Part model, mm, in its own coordinate system. Face numbers are marked on the shaded views. A direction names the side the tool comes from. Round coordinates to 2 decimals unless told otherwise and drop trailing zeros. Loops run counter-clockwise (first coordinate to the right, second up) from the corner with the lowest first, then second, coordinate; pieces in that order, holes last. Notation, with made-up numbers: M 43,29.25 L 89,29.25 A25 ccw 89,65.25 Z; hole C 46,67.5 d5. An arc over 180 degrees is marked long. Put each result on its own line as item: value. Start each with the question number.
```python
from build123d import *

# Parameters (mm, degrees)
SKETCH1_W           = 6.35
SKETCH1_H           = 19.05
SKETCH1_R           = 2.159
BOSS_EXTRUDE1_DEPTH = 19.05
SKETCH2_W           = 14.5796
SKETCH2_H           = 19.05
BOSS_EXTRUDE2_DEPTH = 19.05
SKETCH3_R           = 22.352
CUT_EXTRUDE1_DEPTH  = 2.57175
CUT_EXTRUDE2_REACH  = 34.996
SKETCH4_W           = 3.175
SKETCH4_H           = 19.05
CUT_EXTRUDE3_REACH  = 33.27
SKETCH6_W           = 6.35
SKETCH6_H           = 1.5875
FILLET2_R           = 0.254
FILLET3_START       = -15.6210001
FILLET3_DEPTH       = 5.918275981
FILLET3_START_2     = 9
FILLET3_2_DEPTH     = 8
CUT_EXTRUDE4_START  = -14.5796
CUT_EXTRUDE4_DEPTH  = 14.5796


with BuildPart() as part:
    # Sketch1 → Boss-Extrude1 (new body)
    with BuildSketch(Plane.XY):
        with Locations((3.175, 9.525)):
            Rectangle(SKETCH1_W, SKETCH1_H)
        with Locations(Location((3.175, 14.3764, 0), (0, 0, 180))):
            Circle(SKETCH1_R, mode=Mode.SUBTRACT)
        with Locations(Location((3.175, 4.6736, 0), (0, 0, 180))):
            Circle(SKETCH1_R, mode=Mode.SUBTRACT)
    extrude(amount=BOSS_EXTRUDE1_DEPTH)

    # Sketch2 → Boss-Extrude2 (add)
    with BuildSketch(Plane.ZY):
        with Locations((11.7602, 9.525)):
            Rectangle(SKETCH2_W, SKETCH2_H)
    extrude(amount=BOSS_EXTRUDE2_DEPTH)

    # Sketch3 → Cut-Extrude1 (cut, symmetric)
    with BuildSketch(Plane(origin=(0, 0, 13.31595), x_dir=(-1, 0, 0), z_dir=(0, 0, -1))):
        with Locations((31.4198, 9.525)):
            Circle(SKETCH3_R)
    extrude(amount=CUT_EXTRUDE1_DEPTH, both=True, mode=Mode.SUBTRACT)

    # Cut-Extrude2: up to this face of the body (flat: up to its plane)
    cut_extrude2_end = Plane(part.part.faces().sort_by_distance((3.175, 9.525, 0))[0])
    # Sketch4 → Cut-Extrude2 (cut, up to the picked face)
    with BuildSketch(Plane(origin=(0, 0, 19.05), x_dir=(-1, 0, 0), z_dir=(0, 0, -1)), mode=Mode.PRIVATE) as cut_extrude2_sk1:
        with Locations((17.4625, 9.525)):
            Rectangle(SKETCH4_W, SKETCH4_H)
    cut_extrude2_tool1 = split(extrude(cut_extrude2_sk1.sketch, amount=CUT_EXTRUDE2_REACH, mode=Mode.PRIVATE), bisect_by=cut_extrude2_end, keep=Keep.BOTH, mode=Mode.PRIVATE)
    add(cut_extrude2_tool1.solids().sort_by(Axis((-17.4625, 9.525, 19.05), (0, 0, -1)))[0], mode=Mode.SUBTRACT)

    # Sketch6 → Cut-Extrude3 (cut, up to next)
    with BuildSketch(Plane.XY.offset(19.05), mode=Mode.PRIVATE) as cut_extrude3_sk1:
        with Locations((-12.7, 0.79375)):
            Rectangle(SKETCH6_W, SKETCH6_H)
    cut_extrude3_tool1 = extrude(cut_extrude3_sk1.sketch, amount=-CUT_EXTRUDE3_REACH, mode=Mode.PRIVATE) & part.part
    # Sketch6 → Cut-Extrude3 (cut, up to next)
    with BuildSketch(Plane.XY.offset(19.05), mode=Mode.PRIVATE) as cut_extrude3_sk2:
        with Locations((-12.7, 18.25625)):
            Rectangle(SKETCH6_W, SKETCH6_H)
    cut_extrude3_tool2 = extrude(cut_extrude3_sk2.sketch, amount=-CUT_EXTRUDE3_REACH, mode=Mode.PRIVATE) & part.part
    add(cut_extrude3_tool1.solids().sort_by_distance((-12.7, 0.79375, 19.05))[0], mode=Mode.SUBTRACT)
    add(cut_extrude3_tool2.solids().sort_by_distance((-12.7, 18.25625, 19.05))[0], mode=Mode.SUBTRACT)

    # Fillet2
    fillet2_edges = [part.edges().sort_by_distance(p)[0] for p in [
        (-13.199816574, 1.5875, 10.7442),
        (-15.875, 1.5875, 7.6073),
        (-13.199816574, 1.5875, 15.8877),
        (-15.875, 1.5875, 17.46885),
        (-9.525, 1.5875, 11.7602),
        (-9.525, 0, 11.7602),
        (-13.199816574, 17.4625, 10.7442),
        (-9.525, 19.05, 11.7602),
        (-9.525, 17.4625, 11.7602),
        (-13.199816574, 17.4625, 15.8877),
        (-15.875, 17.4625, 7.6073),
        (-15.875, 17.4625, 17.46885),
        (-15.875, 9.525, 15.8877),
        (-15.875, 9.525, 10.7442),
    ]]
    fillet(fillet2_edges, radius=FILLET2_R)

    # Fillet3: read off the stored shape, not the designer's step
    # Fillet3 outline → Fillet3 (cut)
    with BuildSketch(Plane.YZ.offset(FILLET3_START)):
        with BuildLine():
            ThreePointArc((17.2085, 10.7442), (17.388105122, 10.669805122), (17.4625, 10.4902))
            Line((17.4625, 10.4902), (17.4625, 16.1417))
            ThreePointArc((17.4625, 16.1417), (17.388105122, 15.962094878), (17.2085, 15.8877))
            Line((17.2085, 15.8877), (1.8415, 15.8877))
            ThreePointArc((1.8415, 15.8877), (1.661894878, 15.962094878), (1.5875, 16.1417))
            Line((1.5875, 16.1417), (1.5875, 10.4902))
            ThreePointArc((1.5875, 10.4902), (1.661894878, 10.669805122), (1.8415, 10.7442))
            Line((1.8415, 10.7442), (17.2085, 10.7442))
        make_face()
    extrude(amount=FILLET3_DEPTH, mode=Mode.SUBTRACT)

    # Fillet3 2 outline → Fillet3 2 (add)
    with BuildSketch(Plane.XY.offset(FILLET3_START_2)):
        with BuildLine():
            ThreePointArc((-9.702724219, 4.235338054), (-9.880467378, 2.915439177), (-9.778999483, 1.587497181))
            Line((-9.778999483, 1.587497181), (-9.702724119, 1.5875))
            Line((-9.702724119, 1.5875), (-9.702724219, 4.235338054))
        make_face()
        with BuildLine():
            Line((-9.702724119, 17.4625), (-9.778999483, 17.462502819))
            ThreePointArc((-9.778999483, 17.462502819), (-9.880467378, 16.134560823), (-9.702724219, 14.814661946))
            Line((-9.702724219, 14.814661946), (-9.702724119, 17.4625))
        make_face()
    extrude(amount=FILLET3_2_DEPTH)

    # Cut-Extrude4: read off the stored shape, not the designer's step
    # Cut-Extrude4 outline → Cut-Extrude4 (cut)
    with BuildSketch(Plane.XY.offset(19.05).offset(CUT_EXTRUDE4_START)):
        with BuildLine():
            Line((-9.271, 0), (-3.175, 0))
            Line((-3.175, 0), (-3.175, 3.302))
            Line((-3.175, 3.302), (-9.857519432, 3.302))
            ThreePointArc((-9.857519432, 3.302), (-9.876451593, 2.442083536), (-9.778999483, 1.587497181))
            ThreePointArc((-9.778999483, 1.587497181), (-9.599394878, 1.513105122), (-9.525, 1.3335))
            Line((-9.525, 1.3335), (-9.525, 0.254))
            ThreePointArc((-9.525, 0.254), (-9.450605122, 0.074394878), (-9.271, 0))
        make_face()
        with BuildLine():
            ThreePointArc((-9.778999483, 1.587497181), (-9.876451593, 2.442083536), (-9.857519432, 3.302))
            Line((-9.857519432, 3.302), (-15.875, 3.302))
            Line((-15.875, 3.302), (-15.875, 1.8415))
            ThreePointArc((-15.875, 1.8415), (-15.800605122, 1.661894878), (-15.621, 1.5875))
            Line((-15.621, 1.5875), (-9.778999483, 1.587497181))
        make_face()
    extrude(amount=CUT_EXTRUDE4_DEPTH, mode=Mode.SUBTRACT)


solid = part.part
```
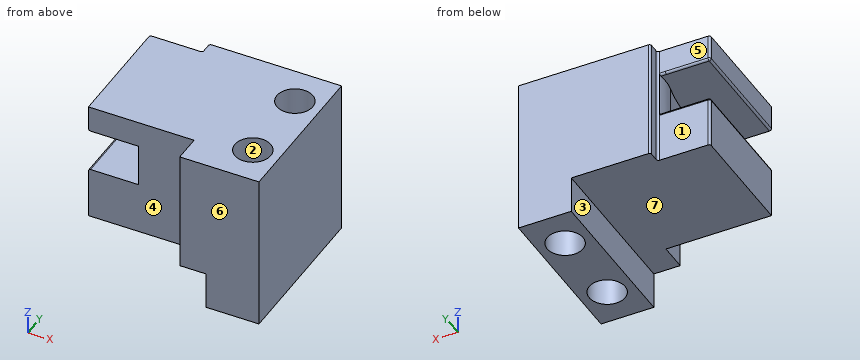
1. Which spindle directions (+Z, -Z, +X, -X, +Y, -Y) get a long thin tool onto all of the face, cutting with end or side? Do the marked faces 5, 6 and 7. Say none if no direction does.
2. Cut at B-B, the plane y = 5. Give the cut face in (x, z) (3 decimals).
3. Cut at D-D, the plane x = 3.5. Give the cut face in (y, z).
4. Wall check: L1, parallel to Z at x = -10, y = 11.75; L2, parallel to Y at x = 3, z = 16.25; L3, parallel to Z at x = -4, y = 6.25. Give the ranges that are in metal, low to high.
5. Cut at C-C, the plane z = 9.75. Give the number of separate pieces and of enclosed holes in the cut face, and give its area (3 significant figures).
6. Drop flat-ended pins along their axis: pin 1 (6.5 mm diameter, centred on x = -12.5, z = 14, fed in from -Y); pin 2 (1.3 mm diameter, centred on y = 7.5, z = 1.5, fed in from -X); pin 3 (3 mm diameter, centred on x = -12, z = 18, fed in from +Y). Give the stop position or say it passes through.
7. Mould opens along Y. For the marked faces 1, 2, 3 and 4 say: released by +Y, released by -Y, zero draft, split by the parting line, or undercut.
8. Cut at A-A, the plane x = -13.75. Give the cut face in (y, z).
Results list:
1. face 5: +Z, -Z, -X, +Y
1. face 6: +Z, -Z, +X, -X, -Y
1. face 7: -Z, -X, +Y, -Y
2. outline: M -15.875,4.47 L 0,4.47 L 0,0 L 1.041,0 L 1.041,19.05 L -15.875,19.05 L -15.875,16.142 A0.254 ccw -15.621,15.888 L -9.531,15.888 L -9.531,10.744 L -15.621,10.744 A0.254 ccw -15.875,10.49 Z; M 5.309,0 L 6.35,0 L 6.35,19.05 L 5.309,19.05 Z
3. outline: M 0,0 L 2.54,0 L 2.54,19.05 L 0,19.05 Z; M 6.81,0 L 12.24,0 L 12.24,19.05 L 6.81,19.05 Z; M 16.51,0 L 19.05,0 L 19.05,19.05 L 16.51,19.05 Z
4. L1: z = 4.47 to 10.74, 15.89 to 19.05
4. L2: y = 0 to 2.52, 6.83 to 12.22, 16.53 to 19.05
4. L3: z = 4.47 to 19.05
5. separate pieces: 1
5. enclosed holes: 2
5. area: 342 mm^2
6. pin 1: stops at y = 3.3
6. pin 2: stops at x = 0
6. pin 3: stops at y = 17.46
7. face 1: released by +Y
7. face 2: undercut
7. face 3: zero draft
7. face 4: released by -Y
8. outline: M 3.3,4.47 L 17.46,4.47 L 17.46,10.49 A0.25 ccw 17.21,10.74 L 3.3,10.74 Z; M 3.3,15.89 L 17.21,15.89 A0.25 ccw 17.46,16.14 L 17.46,19.05 L 3.3,19.05 Z
